Verification items for this drawing (mm, ordinates from the low corner). Round coordinates to 2 decimals unless told otherwise and drop trailing zeros. Loops run counter-clockwise (first coordinate to the right, second up) from the corner with the lowest first, then second, coordinate; pieces in that order, holes last. Notation, with made-up numbers: M 39,-39 L 82,-39 A12 ccw 82,-22 Z; hole C 77,86.5 d10. An arc over 180 degrees is marked long. Answer as CSV lines item,"result".
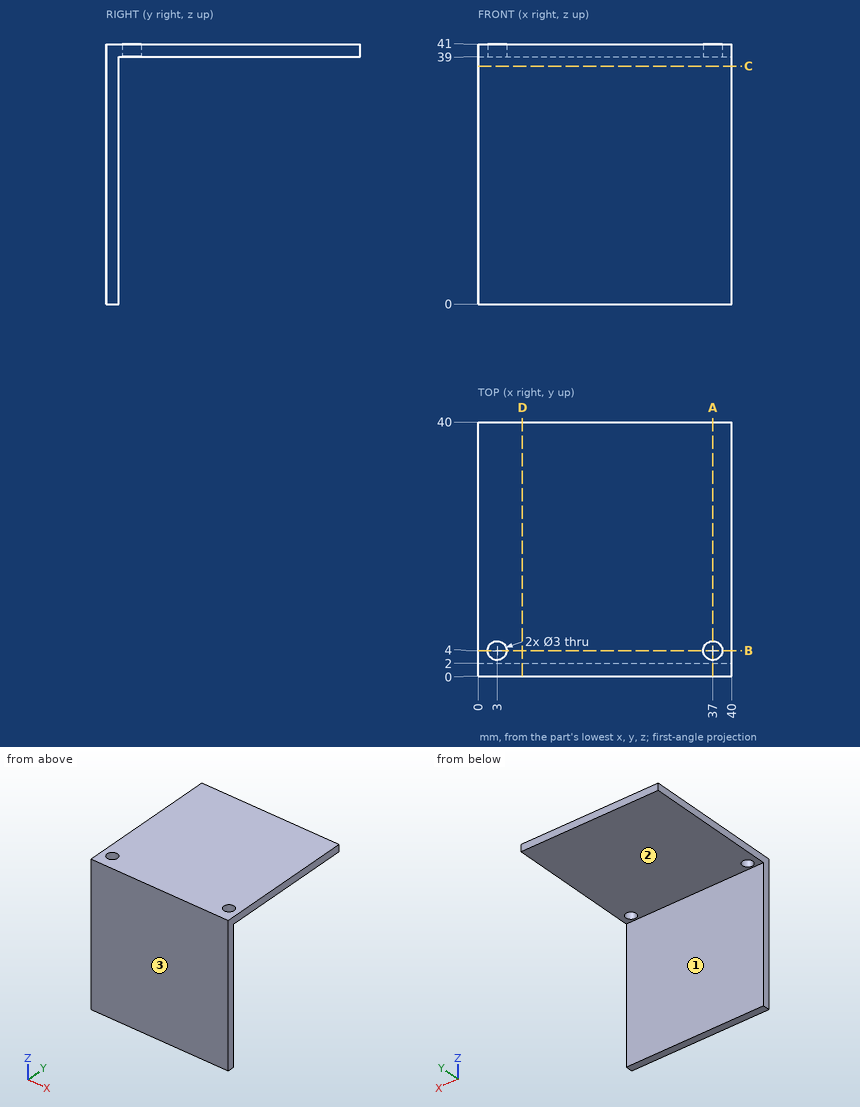
1) Draft check along Y on the marked faces 1, 2 and 3. Enter one of: +Y half, -Y half, draft (parallel to the pull), parting line (faces both ways), or undercut.
Here are the results:
face 1,"+Y half"
face 2,"draft"
face 3,"-Y half"
2) Section check D-D (x = 7). Record the cut outline in (y, z), plus the area to 3 significant figures.
Here are the results:
outline,"M 0,0 L 2,0 L 2,39 L 40,39 L 40,41 L 0,41 Z"
area,"158 mm^2"
3) Go/stop test with flat-tipped pins: pin 1 (3.5 mm diameter, centred on x = 3, y = 4, fed in from -Z); pin 2 (10 mm diameter, centred on y = 10.5, z = 5, fed in from +X); pin 3 (11.5 mm diameter, centred on x = 19, z = 28, fed in from +Y). Record where each tip stops, or that it passes through.
Here are the results:
pin 1,"stops at z = 39"
pin 2,"passes through"
pin 3,"stops at y = 2"
4) Section check B-B (y = 4). Record the cut outline in (x, z), plus the area to 3 significant figures.
Here are the results:
outline,"M 0,39 L 1.5,39 L 1.5,41 L 0,41 Z; M 4.5,39 L 35.5,39 L 35.5,41 L 4.5,41 Z; M 38.5,39 L 40,39 L 40,41 L 38.5,41 Z"
area,"68.0 mm^2"
5) Section check C-C (z = 37.5). Record the cut outline in (x, y).
Here are the results:
outline,"M 0,0 L 40,0 L 40,2 L 0,2 Z"
6) Section check A-A (x = 37). Record the cut outline in (y, z), plus the area to 3 significant figures.
Here are the results:
outline,"M 0,0 L 2,0 L 2,39 L 2.5,39 L 2.5,41 L 0,41 Z; M 5.5,39 L 40,39 L 40,41 L 5.5,41 Z"
area,"152 mm^2"
7) Material ranges on probe 1 along Y at (x, z) = (3, 39.7); probe 2 along Z at (x, y) = (29.5, 17); probe 3 along Y at (x, z) = (21.5, 14), recorded low to high.
Here are the results:
probe 1,"y = 0 to 2.5, 5.5 to 40"
probe 2,"z = 39 to 41"
probe 3,"y = 0 to 2"
